Autodesk Inventor part; units mm, degrees
ref_plane "YZ Plane" through (0, 0, 0) normal (1, 0, 0) x (0, 1, 0)
ref_plane "XZ Plane" through (0, 0, 0) normal (0, 1, 0) x (-1, 0, 0)
ref_plane "XY Plane" through (0, 0, 0) normal (0, 0, 1) x (1, 0, 0)
sketch "Sketch1" plane through (0, 0, 0) normal (0, 1, 0) x (-1, 0, 0)
  line L0 (0, 0) -> (40, 0)
  line L1 (40, 0) -> (40, -80)
  line L2 (40, -80) -> (0, -80)
  line L3 (0, -80) -> (0, 0)
  dimension "d0" = 40
  dimension "d1" = 80
extrude "Extrusion1" add sketch "Sketch1" along normal blind 8
sketch "Sketch2" plane through (0, 8, 0) normal (0, 1, 0) x (1, 0, 0)
  line L0 (-24.4, 15) -> (-15.6, 15)
  line L1 (-15.6, 15) -> (-15.6, 25)
  line L2 (-15.6, 25) -> (-24.4, 25)
  line L3 (-24.4, 25) -> (-24.4, 15)
  line L4 (-40, 0) -> (0, 0)
  line L5 (-24.4, 55) -> (-15.6, 55)
  line L6 (-15.6, 55) -> (-15.6, 65)
  line L7 (-15.6, 65) -> (-24.4, 65)
  line L8 (-24.4, 65) -> (-24.4, 55)
  line L9 (-20, 25) -> (-20, 55) construction
  line L10 (-40, 80) -> (-40, 0) construction
  point P0 (-20, 15)
  point P1 (-20, 0)
  point P2 (-20, 40)
  point P3 (-40, 40)
  dimension "d4" = 8.8
  dimension "d5" = 10
  dimension "d6" = 10
  dimension "d7" = 8.8
  dimension "d8" = 30
extrude "Extrusion2" add sketch "Sketch2" along normal blind 14
fillet "Fillet1" radius 5 4 edges at (-20, 22, -15) (-20, 22, -25) (-20, 22, -55) (-20, 22, -65)
sketch "Sketch3" plane through (-15.6, 8, -15) normal (1, 0, 0) x (0, 0, -1)
  arc A0 (10, 9) -> (0, 9) centre (5, 9) ccw
  circle A1 centre (5, 9) radius 1
  arc A2 (50, 9) -> (40, 9) centre (45, 9) ccw
  circle A3 centre (45, 9) radius 1
  point P0 (-15, -8)
  dimension "d12" = 2
  dimension "d13" = 2
extrude "Extrusion3" cut sketch "Sketch3" against normal blind 14
sketch "Sketch4" plane through (-40, 0, 0) normal (0, 0, 1) x (1, 0, 0)
  circle A0 centre (20, 4) radius 1
  line L0 (40, 0) -> (40, 8)
  line L1 (0, 8) -> (40, 8)
  point P0 (40, 4)
  point P1 (20, 8)
  dimension "d16" = 2
extrude "Extrusion4" cut sketch "Sketch4" against normal blind 5
sketch "Sketch5" plane through (0, 0, -80) normal (0, 0, -1) x (-1, 0, 0)
  circle A0 centre (20, 4) radius 1
  point P0 (0, 0)
extrude "Extrusion5" cut sketch "Sketch5" against normal blind 5
sketch "Sketch6" plane through (0, 8, 0) normal (0, 1, 0) x (1, 0, 0)
  line L0 (-27.5, 50) -> (-12.5, 50)
  line L1 (-12.5, 50) -> (-12.5, 30)
  line L2 (-12.5, 30) -> (-27.5, 30)
  line L3 (-27.5, 30) -> (-27.5, 50)
  line L4 (-40, 80) -> (-40, 0)
  line L5 (-40, 0) -> (0, 0)
  point P0 (-12.5, 40)
  point P1 (-40, 40)
  point P2 (-20, 50)
  point P3 (-20, 0)
  dimension "d21" = 20
  dimension "d22" = 15
extrude "Extrusion6" cut sketch "Sketch6" against normal up to surface (8 mm away)
properties part number "basePlate"
Design review of the part built by this model. Coordinates are the model's own, in mm. A direction names the side the tool comes from. Round coordinates to 2 decimals unless told otherwise and drop trailing zeros. Write each loop counter-clockwise with the first axis right and the second up, starting at its lowest first coordinate (ties: lowest second). Pieces come first, ordered by that corner, then holes.
Item 1: We need section D-D on z = -13. Write out the cut boundary in (x, y), and give its area (3 significant figures).
Item 2: We need section B-B on y = 12.5. Write out the cut boundary in (x, z).
Item 3: Clearance check with flat-ended pins moving along their axes: pin 1 Ø4.5 at (x, y) = (-22, 10.5) entering from +Z; pin 2 Ø5 at (x, z) = (-5.5, -14) entering from +Y; pin 3 Ø11 at (y, z) = (15.5, -20) entering from -X; pin 4 Ø1.6 at (y, z) = (17, -20) entering from +X. State where each tip first meets the part, or that it passes through.
Item 4: We need section A-A on x = -20. State how many separate pieces and enclosed holes the cut face has, and give its area (3 significant figures).
Item 5: We need section C-C on z = -44. Write out the cut boundary in (x, y).
Item 6: For faces 5 (the flat face through (-20, 12, -55)), 6 (the flat face through (-20, 12, -65)), 7 (the flat face through (-15.6, 15, -60)), 8 (the cylindrical face through (-20.737, 4.676, -2.465)), 9 (the flat face through (-12.5, 4, -40)), list the 3-axis set-ups (+Z, -Z, +X, -X, +Y, -Y) from which the entire face can be reached by the end or side of a thin tool; tool diameter is ignored.
Item 7: For probe 1 along Z at (x, y) = (-15.5, 1.5); probe 2 along Z at (x, y) = (-19, 13.25); probe 3 along Y at (x, z) = (-18.75, -60), list the stretches that pass through material, from the lowest coordinate up.
Item 8: The part is to be moulded in two halves that separate along Y. For faces 1 (the flat face through (-20, 12, -25)), 2 (the cylindrical face through (-20, 16, -20)), 3 (the flat face through (-29, 0, -39)), 4 (the cylindrical face through (-20, 21, -23)), say which applies: +Y half, -Y half, draft (parallel to the pull), parting line (faces both ways), or undercut.
Returned:
1. outline: (-40, 0) - (0, 0) - (0, 8) - (-40, 8) - close
1. area: 320 mm2
2. outline: (-24.4, -65) - (-15.6, -65) - (-15.6, -55) - (-24.4, -55) - close; (-24.4, -25) - (-15.6, -25) - (-15.6, -15) - (-24.4, -15) - close
3. pin 1: stops at z = -15
3. pin 2: stops at y = 8
3. pin 3: stops at x = -24.4
3. pin 4: passes through
4. separate pieces: 2
4. enclosed holes: 2
4. area: 712 mm2
5. outline: (-40, 0) - (-27.5, 0) - (-27.5, 8) - (-40, 8) - close; (-12.5, 0) - (0, 0) - (0, 8) - (-12.5, 8) - close
6. face 5: +X, -X, +Y
6. face 6: -Z, +X, -X, +Y
6. face 7: +Z, -Z, +X, +Y
6. face 8: +Z
6. face 9: +Y, -Y
7. probe 1: z = -80 to -50, -30 to 0
7. probe 2: z = -65 to -55, -25 to -15
7. probe 3: y = 0 to 16, 18 to 22
8. face 1: draft
8. face 2: undercut
8. face 3: -Y half
8. face 4: +Y half
